Build history of the part. All positions in model axes, mm. A direction names the side the tool comes from. Give positions to 0.01 mm unless a question says otherwise; leave off trailing zeros. Loops run counter-clockwise (first coordinate to the right, second up) from the corner with the lowest first, then second, coordinate; pieces in that order, holes last. Notation, with made-up numbers: M 46.25,63.5 L 87.25,63.5 A14 ccw 87.25,75.5 Z; hole C -10.75,88.25 d8. An arc over 180 degrees is marked long. Put each result on its own line as item: value.
```python
from build123d import *

# Parameters (mm, degrees)
SKETCH1_R               = 50
SKETCH1_R_2             = 47.5
BOSS_EXTRUDE1_DEPTH     = 10
SKETCH2_R               = 50
BOSS_EXTRUDE2_DEPTH     = 30
SKETCH4_R               = 2.5
SKETCH6_R               = 50
CUT_EXTRUDE2_DEPTH      = 3
CUT_EXTRUDE3_DEPTH      = 80.806014811
CUT_EXTRUDE3_DEPTH_BACK = 80.806014811
SKETCH7_R               = 2.5
FILLET1_R               = 10
SKETCH9_R               = 25
CUT_EXTRUDE5_DEPTH      = 10


with BuildPart() as part:
    # Sketch1 → Boss-Extrude1 (new body)
    with BuildSketch(Plane(origin=(0, 0, 0), x_dir=(1, 0, 0), z_dir=(0, 1, 0))):
        with Locations(Location((0, 0, 0), (0, 0, 270))):
            Circle(SKETCH1_R)
        with Locations(Location((0, 0, 0), (0, 0, 270))):
            Circle(SKETCH1_R_2, mode=Mode.SUBTRACT)
    extrude(amount=BOSS_EXTRUDE1_DEPTH)

    # Sketch2 → Boss-Extrude2 (add)
    with BuildSketch(Plane(origin=(0, 10, 0), x_dir=(1, 0, 0), z_dir=(0, 1, 0))):
        with Locations(Location((0, 0, 0), (0, 0, 270))):
            Circle(SKETCH2_R)
    extrude(amount=BOSS_EXTRUDE2_DEPTH)

    # Cut-Sweep1: sweep along a path in Sketch3
    with BuildLine(Plane.XZ.offset(-10)) as cut_sweep1_path:
        CenterArc((0, 0), 42.5, 0, 360)
    # Sketch4 → Cut-Sweep1 (sweep, cut)
    with BuildSketch(Plane.XY):
        with Locations((42.5, 10)):
            Circle(SKETCH4_R)
    sweep(path=cut_sweep1_path.line, mode=Mode.SUBTRACT)

    # Sketch6 → Cut-Extrude2 (cut)
    with BuildSketch(Plane.XZ):
        with Locations(Location((0, 0, 0), (0, 0, 270))):
            Circle(SKETCH6_R)
    extrude(amount=-CUT_EXTRUDE2_DEPTH, mode=Mode.SUBTRACT)

    # Sketch7 → Cut-Extrude3 (cut, two sides: drawn at the far end of the back side and taken through both)
    with BuildSketch(Plane(origin=(0, 40, 0), x_dir=(1, 0, 0), z_dir=(0, 1, 0)).offset(-CUT_EXTRUDE3_DEPTH_BACK)):
        with Locations(Location((0, 0, 0), (0, 0, 270))):
            Circle(SKETCH7_R)
    extrude(amount=CUT_EXTRUDE3_DEPTH + CUT_EXTRUDE3_DEPTH_BACK, mode=Mode.SUBTRACT)

    # Fillet1
    fillet1_edges = [part.edges().sort_by_distance(p)[0] for p in [
        (0, 40, -50),
    ]]
    fillet(fillet1_edges, radius=FILLET1_R)

    # Sketch9 → Cut-Extrude5 (cut)
    with BuildSketch(Plane(origin=(0, 40, 0), x_dir=(1, 0, 0), z_dir=(0, 1, 0))):
        with Locations(Location((0, 0, 0), (0, 0, 270))):
            Circle(SKETCH9_R)
    extrude(amount=-CUT_EXTRUDE5_DEPTH, mode=Mode.SUBTRACT)


solid = part.part
```
Q1. Mould opens along Z. For faces 1 (the cylindrical face through (15.02, 16.31, 47.69)), 2 (the flat face through (-17, 10, 42)), 3 (the flat face through (-18.3, 3, -44.2)) say: pulls with the +Z half, pulls with the -Z half, needs draft (parallel to the pull), parting line crosses it, or undercut.
Here are the results:
face 1: parting line crosses it
face 2: undercut
face 3: needs draft
Q2. Probe line 1 (X direction, y = 17.5, z = 0); line 2 (X direction, y = 12, z = -23); line 3 (X direction, y = 8.5, z = 0). List the from-to ranges inside material, lowest first. Write a range as from..to.
Here are the results:
line 1: -50..-2.5, 2.5..50
line 2: -44.4..-37.51, -33.94..33.94, 37.51..44.4
line 3: -50..-47.5, 47.5..50
Q3. Drop flat-ended pins along their axis: pin 1 Ø1 at (x, z) = (-6, 25) entering from -Y; pin 2 Ø6 at (y, z) = (32, 13.5) entering from -X; pin 3 Ø2 at (y, z) = (11, -11) entering from +X. Give the stop position or say it passes through.
Here are the results:
pin 1: y = 10
pin 2: x = -48.8
pin 3: x = 48.99
Q4. Slice it at B-B (z = 0). List the corners of the cut face in (x, y), and give its area (3 significant figures).
Here are the results:
outline: M -50,3 L -47.5,3 L -47.5,10 L -45,10 A2.5 cw -40,10 L -2.5,10 L -2.5,30 L -25,30 L -25,40 L -40,40 A10 ccw -50,30 Z; M 2.5,10 L 40,10 A2.5 cw 45,10 L 47.5,10 L 47.5,3 L 50,3 L 50,30 A10 ccw 40,40 L 25,40 L 25,30 L 2.5,30 Z
area: 2,370 mm²
Q5. Slice it at A-A (x = 0). List the corners of the cut face in (y, z).
Here are the results:
outline: M 3,-50 L 30,-50 A10 ccw 40,-40 L 40,-25 L 30,-25 L 30,-2.5 L 10,-2.5 L 10,-40 A2.5 cw 10,-45 L 10,-47.5 L 3,-47.5 Z; M 3,47.5 L 10,47.5 L 10,45 A2.5 cw 10,40 L 10,2.5 L 30,2.5 L 30,25 L 40,25 L 40,40 A10 ccw 30,50 L 3,50 Z
Q6. Tool access for faces 4 (the cylindrical face through (7.509, 35.07, 23.846)), 5 (the cylindrical face through (-2.44, 19.86, -0.54)), 6 (the flat face through (1, 10, 8)): list every direction of +Z, -Z, +X, -X, +Y, -Y with a clear straight run to the whole face (end or side of a thin tool).
Here are the results:
face 4: +Y
face 5: +Y, -Y
face 6: -Y
Q7. Slice it at C-C (y = 19.5). List the corners of the cut face in (x, z).
Here are the results:
outline: C 0,0 d100; hole C 0,0 d5
